from build123d import *
from OCP.BRepFilletAPI import BRepFilletAPI_MakeChamfer

# Parameters (mm, degrees)
BOSS_EXTRUDE1_DEPTH      = 0.85
SKETCH3_R                = 0.5
BOSS_EXTRUDE2_DEPTH      = 0.65
SKETCH4_W                = 6.9
SKETCH4_H                = 1.9
BOSS_EXTRUDE3_DEPTH      = 0.4
FILLET1_R                = 0.4
CHAMFER1_SIZE            = 1.2
CHAMFER1_SIZE2           = 0.3
FILLET2_R                = 0.4
BOSS_EXTRUDE4_DEPTH      = 0.2
BOSS_EXTRUDE4_DEPTH_BACK = 1.4
SKETCH7_R                = 0.4
BOSS_EXTRUDE5_DEPTH      = 0.2
BOSS_EXTRUDE5_DEPTH_BACK = 1.4
SKETCH8_R                = 0.4
SKETCH6_W                = 0.5
SKETCH6_H                = 1.7
CUT_EXTRUDE1_DEPTH       = 11.940292501
SKETCH9_R                = 0.35
BOSS_EXTRUDE6_DEPTH      = 0.1
SKETCH10_R               = 0.3
BOSS_EXTRUDE7_DEPTH      = 0.8
SCALE1_SCALE             = 2


with BuildPart() as part:
    # Sketch1 → Boss-Extrude1 (new, symmetric)
    with BuildSketch(Plane(origin=(0, 0, 0), x_dir=(1, 0, 0), z_dir=(0, 1, 0))):
        Polygon((-3.35, 0), (-3.35, 10.1), (3.35, 10.1), (3.35, 0), (3.6, 0), (3.6, -2.4), (2.3, -2.4), (2.3, 0), (2.55, 0), (2.55, 8.7), (-2.55, 8.7), (-2.55, 0), (-2.3, 0), (-2.3, -2.4), (-3.6, -2.4), (-3.6, 0), align=None)
    extrude(amount=BOSS_EXTRUDE1_DEPTH, both=True)

    # Sketch3 → Boss-Extrude2 (add, symmetric)
    # profile 1 of 2: a face of its own
    with BuildSketch(Plane(origin=(0, 0, 0), x_dir=(1, 0, 0), z_dir=(0, 1, 0))):
        Polygon((-0.75, 8.7), (-2.55, 8.7), (-2.55, 3.2), align=None)
        with Locations(Location((-2, 7.9, 0), (0, 0, 270))):
            Circle(SKETCH3_R, mode=Mode.SUBTRACT)
    # profile 2 of 2: a face of its own
    with BuildSketch(Plane(origin=(0, 0, 0), x_dir=(1, 0, 0), z_dir=(0, 1, 0))):
        Polygon((2.55, 3.2), (0.75, 8.7), (2.55, 8.7), align=None)
        with Locations(Location((2, 7.9, 0), (0, 0, 90))):
            Circle(SKETCH3_R, mode=Mode.SUBTRACT)
    extrude(amount=BOSS_EXTRUDE2_DEPTH, both=True)

    # Sketch4 → Boss-Extrude3 (add)
    with BuildSketch(Plane(origin=(0, 0, -10.1), x_dir=(-1, 0, 0), z_dir=(0, 0, -1))):
        Rectangle(SKETCH4_W, SKETCH4_H)
    extrude(amount=-BOSS_EXTRUDE3_DEPTH)

    # Fillet1
    fillet1_edges = [part.edges().sort_by_distance(p)[0] for p in [
        (2.95, -0.85, 2.4),
        (-2.95, -0.85, 2.4),
    ]]
    fillet(fillet1_edges, radius=FILLET1_R)

    # Chamfer1: one chamfer whose edges measure the first distance from different faces: ONE call of the kernel's chamfer builder (chamfer() names one face for all edges)
    chamfer1_edges_1 = [part.edges().sort_by_distance(p)[0] for p in [
        (-2.95, 0.85, 2.4),
    ]]
    chamfer1_side_1 = [part.faces().sort_by_distance(p)[0] for p in [
        (-2.95, 0.2, 2.4),
    ]]
    chamfer1_edges_2 = [part.edges().sort_by_distance(p)[0] for p in [
        (2.95, 0.85, 2.4),
    ]]
    chamfer1_side_2 = [part.faces().sort_by_distance(p)[0] for p in [
        (2.95, 0.2, 2.4),
    ]]
    chamfer1 = BRepFilletAPI_MakeChamfer(part.part.solid().wrapped)
    for e in chamfer1_edges_1:
        chamfer1.Add(CHAMFER1_SIZE, CHAMFER1_SIZE2, e.wrapped, chamfer1_side_1[0].wrapped)  # the first distance lies on this face
    for e in chamfer1_edges_2:
        chamfer1.Add(CHAMFER1_SIZE, CHAMFER1_SIZE2, e.wrapped, chamfer1_side_2[0].wrapped)  # the first distance lies on this face
    add(Compound.cast(chamfer1.Shape()), mode=Mode.REPLACE)

    # Fillet2
    fillet2_edges = [part.edges().sort_by_distance(p)[0] for p in [
        (-2.95, 0.85, 2.1),
        (2.95, 0.85, 2.1),
    ]]
    fillet(fillet2_edges, radius=FILLET2_R)

    # Sketch7 → Boss-Extrude4 (add, two sides: drawn at the far end of the back side and taken through both)
    with BuildSketch(Plane.ZY.offset(3.6).offset(-BOSS_EXTRUDE4_DEPTH_BACK)):
        with Locations((1.9, -0.35)):
            Circle(SKETCH7_R)
    extrude(amount=BOSS_EXTRUDE4_DEPTH + BOSS_EXTRUDE4_DEPTH_BACK)

    # Sketch8 → Boss-Extrude5 (add, two sides: drawn at the far end of the back side and taken through both)
    with BuildSketch(Plane(origin=(3.6, 0, 0), x_dir=(0, 0, -1), z_dir=(1, 0, 0)).offset(-BOSS_EXTRUDE5_DEPTH_BACK)):
        with Locations(Location((-1.9, -0.35, 0), (0, 0, 180))):
            Circle(SKETCH8_R)
    extrude(amount=BOSS_EXTRUDE5_DEPTH + BOSS_EXTRUDE5_DEPTH_BACK)

    # Sketch6 → Cut-Extrude1 (cut, through all)
    with BuildSketch(Plane(origin=(0, 0.85, 0), x_dir=(1, 0, 0), z_dir=(0, 1, 0))):
        with Locations((-2.95, -1.55)):
            Rectangle(SKETCH6_W, SKETCH6_H)
        with Locations((2.95, -1.55)):
            Rectangle(SKETCH6_W, SKETCH6_H)
    extrude(amount=-CUT_EXTRUDE1_DEPTH, mode=Mode.SUBTRACT)

    # Sketch9 → Boss-Extrude6 (add)
    with BuildSketch(Plane.XZ.offset(0.85)):
        with Locations(Location((-2.9, -9.25, 0), (0, 0, 90))):
            Circle(SKETCH9_R)
        with Locations(Location((2.9, -9.25, 0), (0, 0, 90))):
            Circle(SKETCH9_R)
    extrude(amount=BOSS_EXTRUDE6_DEPTH)

    # Sketch10 → Boss-Extrude7 (add)
    with BuildSketch(Plane(origin=(0, 0.85, 0), x_dir=(1, 0, 0), z_dir=(0, 1, 0))):
        with Locations(Location((-2.9, 9.25, 0), (0, 0, 270))):
            Circle(SKETCH10_R)
        with Locations(Location((2.9, 9.25, 0), (0, 0, 270))):
            Circle(SKETCH10_R)
    extrude(amount=BOSS_EXTRUDE7_DEPTH)


with BuildPart() as part_1:
    # Scale1: scaled about (0, 0, 0)
    add(part.part.scale(SCALE1_SCALE))


solid = part_1.part
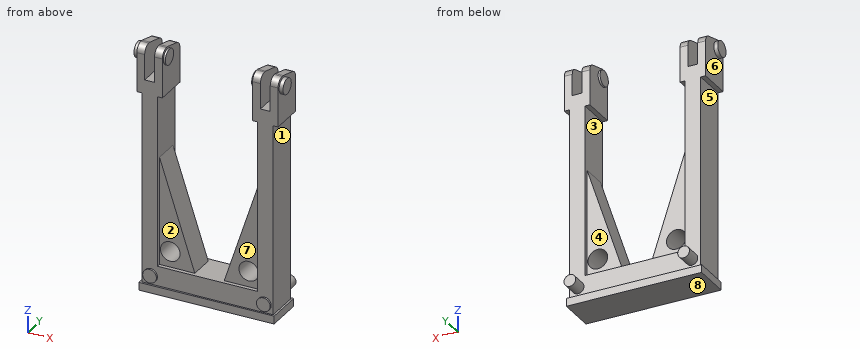
Work out the finished part from the listing and answer in its coordinate system (mm). Face numbers are marked on the shaded views. A direction names the side the tool comes from. Round coordinates to 2 decimals unless told otherwise and drop trailing zeros. Write each loop counter-clockwise with the first axis right and the second up, starting at its lowest first coordinate (ties: lowest second). Pieces come first, ordered by that corner, then holes. Notation, with made-up numbers: (4.25, 89.5) -> (50.25, 89.5) arc R18 ccw to (50.25, 122.5) -> close; hole circle Ø6 at (-4.75, 12.25). An arc over 180 degrees is marked (long way). Write each question's results on one line, items separated by ' | '.
Item 1: Find the intervals of material crossed by line 1 along X through (y, z) = (0.3, -15.8); line 2 along X through (y, z) = (1.25, -4.25); line 3 along X through (y, z) = (-0.2, -15.5), in increasing order. Write a range as [from, to].
Result set:
line 1: [-6.7, -5], [-3, -2.02], [2.02, 3], [5, 6.7] | line 2: [-6.7, -5.1], [5.1, 6.7] | line 3: [-6.7, -4.95], [-3.05, -2.12], [2.12, 3.05], [4.95, 6.7]
Item 2: The mould has two halves that part along Z. Classify the marked faces 6, 7 and 8: +Z half, -Z half, draft (parallel to the pull), parting line (faces both ways), or undercut.
Result set:
face 6: draft | face 7: undercut | face 8: -Z half
Item 3: A cutting plane is placed at C-C, the plane z = -18.5. Determine the outline of the cut face in (x, y), plus the area to 3 significant figures.
Result set:
outline: (-6.7, -1.7) -> (-6.5, -1.7) -> (-6.5, -1.9) -> (-5.1, -1.9) -> (-5.1, -1.7) -> (5.1, -1.7) -> (5.1, -1.9) -> (6.5, -1.9) -> (6.5, -1.7) -> (6.7, -1.7) -> (6.7, 1.7) -> (6.4, 1.7) -> (6.4, 3.3) -> (5.2, 3.3) -> (5.2, 1.7) -> (-5.2, 1.7) -> (-5.2, 3.3) -> (-6.4, 3.3) -> (-6.4, 1.7) -> (-6.7, 1.7) -> close | area: 50.0 mm^2
Item 4: A cutting plane is placed at A-A, the plane z = -0.75. Determine the outline of the cut face in (x, y).
Result set:
outline: (-6.7, -1.7) -> (-5.1, -1.7) -> (-5.1, 1.7) -> (-6.7, 1.7) -> close; (5.1, -1.7) -> (6.7, -1.7) -> (6.7, 1.7) -> (5.1, 1.7) -> close
Item 5: A cutting plane is placed at B-B, the plane x = -5.8. Determine the outline of the cut face in (y, z).
Result set:
outline: (-1.9, -20.2) -> (1.9, -20.2) -> (1.9, -19.4) -> (1.7, -19.4) -> (1.7, -19.1) -> (3.3, -19.1) -> (3.3, -17.9) -> (1.7, -17.9) -> (1.7, 1.4) -> (-1.7, 1.4) -> (-1.7, -17.8) -> (-1.9, -17.8) -> (-1.9, -19.2) -> (-1.7, -19.2) -> (-1.7, -19.4) -> (-1.9, -19.4) -> close
Item 6: Flat-ended cylindrical pins translate along their axes: P1, Ø2, axis at y = 2.5, z = -17.5, coming from the +X side; P2, Ø1.8, axis at x = -3, z = -11, coming from the +Y side; P3, Ø1.5, axis at x = -3.5, z = -7, coming from the +Y side; P4, Ø0.6, axis at x = 2.5, z = -20, coming from the +Y side. Find the tip coordinate at first contact, or state that the pin passes through.
Result set:
P1: x = 6.7 | P2: y = 1.3 | P3: through | P4: y = 1.9
Item 7: A cutting plane is placed at D-D, the plane x = 3.25. Determine the outline of the cut face in (y, z), plus the area to 3 significant figures.
Result set:
outline: (-1.9, -20.2) -> (1.9, -20.2) -> (1.9, -19.4) -> (1.7, -19.4) -> (1.7, -17.4) -> (1.3, -17.4) -> (1.3, -16.46) -> (-1.3, -16.46) -> (-1.3, -17.4) -> (-1.7, -17.4) -> (-1.7, -19.4) -> (-1.9, -19.4) -> close; (-1.3, -15.14) -> (1.3, -15.14) -> (1.3, -12.05) -> (-1.3, -12.05) -> close | area: 20.3 mm^2
Item 8: Which of the six approach directions +Z, -Z, +X, -X, +Y, -Y give full straight-line access (tool end or side, diameter ignored) to the marked faces 1, 2, 3, 4 and 5?
Result set:
face 1: +X, +Y, -Y | face 2: -Y | face 3: none | face 4: +Y | face 5: -X, +Y, -Y
